Answer from the drawing. Dimensions are ordinates in mm from the lowest x, y and z of the part. A direction names the side the tool comes from. Give positions to 0.01 mm unless a question says otherwise; leave off trailing zeros. Order: outer loops, then holes, each group sorted by start corner. A loop starts at its lowest first (then second) coordinate and runs counter-clockwise, first axis right, second up. Notation, with made-up numbers: (-14.5, 53.5) - (29.5, 53.5) arc R22 cw to (29.5, 77.5) - close; hole circle Ø5 at (36, 17). An arc over 180 degrees is marked (long way). Answer in a Markdown table with one row per item.
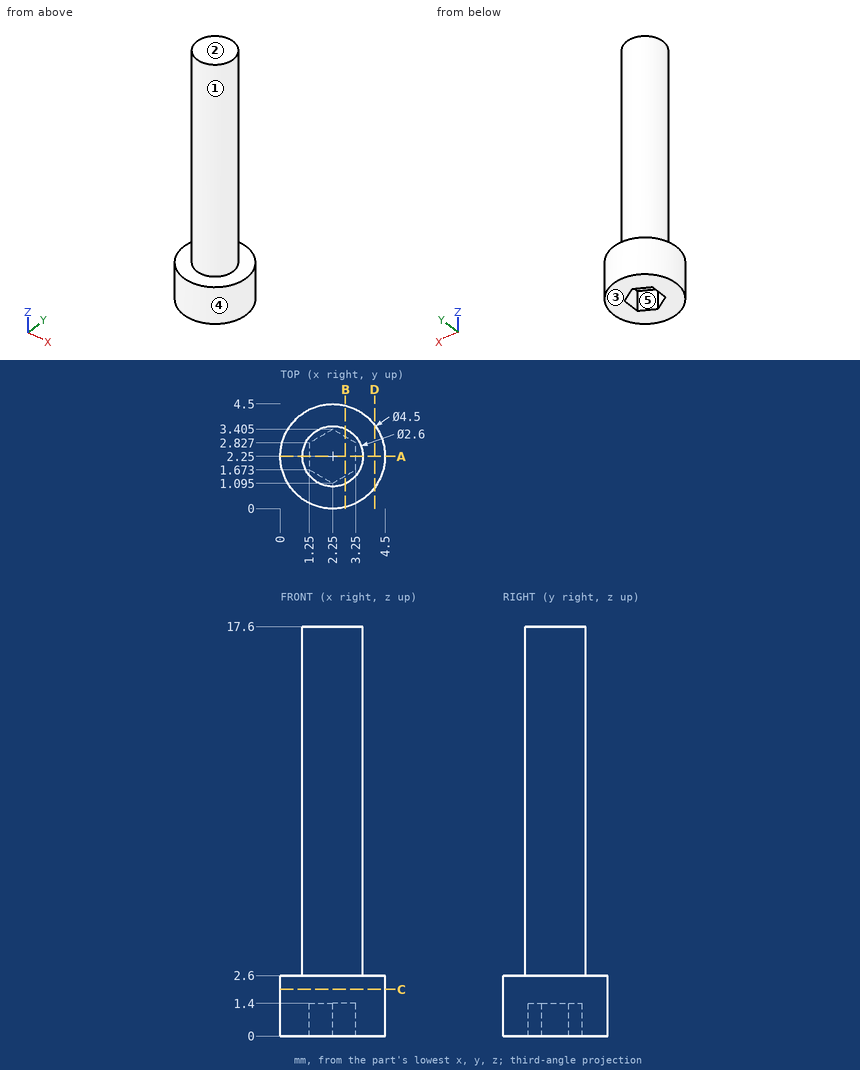
Item 1: Find section D-D on x = 4.05. Write down the section's boundary in (y, z).
Answer block:
| item | result |
|---|---|
| outline | (0.9, 0) - (3.6, 0) - (3.6, 2.6) - (0.9, 2.6) - close |
Item 2: Which of the six approach directions +Z, -Z, +X, -X, +Y, -Y give full straight-line access (tool end or side, diameter ignored) to the marked faces 1 and 2?
Answer block:
| item | result |
|---|---|
| face 1 | +Z |
| face 2 | +Z, +X, -X, +Y, -Y |
Item 3: Find section C-C on z = 2. Write down the section's boundary in (x, y), then the cut area to 3 significant figures.
Answer block:
| item | result |
|---|---|
| outline | circle Ø4.5 at (2.25, 2.25) |
| area | 15.9 mm² |
Item 4: Each of these flat-tipped pins is pushed along its axis until it touches: P1, Ø1.5, axis at x = 3.5, z = 13, coming from the +Y side; P2, Ø1, axis at y = 2, z = 5, coming from the +X side; P3, Ø2, axis at x = 3, z = 5.5, coming from the +Y side. Where does it stop, or does it pass through?
Answer block:
| item | result |
|---|---|
| P1 | y = 3.45 |
| P2 | x = 3.55 |
| P3 | y = 3.55 |
Item 5: Determine the mould class of the marked faces 3, 4 and 5 for opening direction X: pulls with the +X half, pulls with the -X half, needs draft (parallel to the pull), parting line crosses it, or undercut.
Answer block:
| item | result |
|---|---|
| face 3 | needs draft |
| face 4 | parting line crosses it |
| face 5 | undercut |
Item 6: Find section B-B on x = 2.8. Write down the section's boundary in (y, z).
Answer block:
| item | result |
|---|---|
| outline | (0.07, 0) - (1.41, 0) - (1.41, 1.4) - (3.09, 1.4) - (3.09, 0) - (4.43, 0) - (4.43, 2.6) - (3.43, 2.6) - (3.43, 17.6) - (1.07, 17.6) - (1.07, 2.6) - (0.07, 2.6) - close |
Item 7: Find section A-A on y = 2.25. Write down the section's boundary in (x, z).
Answer block:
| item | result |
|---|---|
| outline | (0, 0) - (1.25, 0) - (1.25, 1.4) - (3.25, 1.4) - (3.25, 0) - (4.5, 0) - (4.5, 2.6) - (3.55, 2.6) - (3.55, 17.6) - (0.95, 17.6) - (0.95, 2.6) - (0, 2.6) - close |
Item 8: Consider line 1 (Z direction, x = 4, y = 1.25); line 2 (Z direction, x = 1.6, y = 1.55); line 3 (X direction, y = 4.15, z = 2.25) (1 decimal). Determine where each line is inside the solid, lowest interval first.
Answer block:
| item | result |
|---|---|
| line 1 | 0 to 2.6 |
| line 2 | 1.4 to 17.6 |
| line 3 | 1 to 3.5 |
